Source: CAD feature listing. Evaluate the final solid. Frame: model axes, mm. A direction names the side the tool comes from. Coordinates: 2 decimals unless noted, no trailing zeros. Order: outer loops, then holes, each group sorted by start corner. A loop starts at its lowest first (then second) coordinate and runs counter-clockwise, first axis right, second up. Notation, with made-up numbers: (0.5, 14.5) - (44.5, 14.5) arc R9 cw to (44.5, 25.5) - close; hole circle Ø8 at (38, -21.5). An arc over 180 degrees is marked (long way). One line per question, with ' | ' between items. Start each with the question number.
(1) Contact query for flat-ended pins moving along their axis: P1, Ø5, axis at x = -55.5, z = 10.5, coming from the -Y side; P2, Ø5, axis at x = 1.5, z = -20, coming from the +Y side; P3, Ø8, axis at x = 1.5, z = 20, coming from the -Y side; P4, Ø3, axis at x = -48.5, z = -20, coming from the +Y side. Output: stop coordinate, or through.
(2) Line query: line 1 along X through (y, z) = (22.05, 20); line 2 along X through (y, z) = (8.25, 18.5); line 3 along Z through (x, y) = (51.5, 12.75). Output: solid intervals per line, ascending.
(3) Draft query along Z for faces 5 (the flat face through (1, 15, -33)), 6 (the flat face through (1, 8, 31.2)), 7 (the flat face through (1, 24.25, 0)). Return one class per face: +Z half, -Z half, draft (parallel to the pull), parting line (faces both ways), or undercut.
(4) Section B-B (z = 9.92). Return the cut outline in (x, y), then the cut area to 3 significant figures.
(5) Section A-A (x = -24). Return the cut outline in (y, z), then the cut area to 3 significant figures.
(6) Section C-C (z = 20). Count the separate pieces of the cut face and the enclosed holes in it, then the cut area to 3 significant figures.
(7) Access query for faces 1 (the cylindrical face through (-56.542, 11.694, -5.981)), 2 (the flat face through (40, 21.05, -19)), 3 (the flat face through (-57.7, 8, 2)), 4 (the cylindrical face through (39.94, 17.82, -20.35)). Directions: +Z, -Z, +X, -X, +Y, -Y. A direction counts if a zero-diameter tool reaches every point of the face in a straight line with its end or side. Return the directions, or none.
from build123d import *

# Parameters (mm, degrees)
SKETCH1_W           = 107
SKETCH1_H           = 54
BOSS_EXTRUDE1_DEPTH = 13
CUT_EXTRUDE1_DEPTH  = 2.2
BOSS_EXTRUDE2_DEPTH = 4
FILLET1_R           = 2
SKETCH4_R           = 6
CUT_EXTRUDE2_DEPTH  = 6
CUT_EXTRUDE3_DEPTH  = 6
SKETCH9_R           = 4
SKETCH9_R_2         = 1.6
BOSS_EXTRUDE3_DEPTH = 9.75
SKETCH10_R          = 3
CUT_EXTRUDE5_DEPTH  = 3.2
SKETCH10_3_R        = 1.6
CUT_EXTRUDE6_DEPTH  = 71.13023599


with BuildPart() as part:
    # Sketch1 → Boss-Extrude1 (new body)
    with BuildSketch(Plane(origin=(0, 7.25, 0), x_dir=(1, 0, 0), z_dir=(0, 1, 0))):
        with BuildLine():
            Line((-54.5, -33), (54.5, -33))
            ThreePointArc((54.5, -33), (58.035533906, -31.535533906), (59.5, -28))
            Line((59.5, -28), (59.5, 28))
            ThreePointArc((59.5, 28), (58.035533906, 31.535533906), (54.5, 33))
            Line((54.5, 33), (-54.5, 33))
            ThreePointArc((-54.5, 33), (-58.035533906, 31.535533906), (-59.5, 28))
            Line((-59.5, 28), (-59.5, -28))
            ThreePointArc((-59.5, -28), (-58.035533906, -31.535533906), (-54.5, -33))
        make_face()
        Rectangle(SKETCH1_W, SKETCH1_H, mode=Mode.SUBTRACT)
    extrude(amount=BOSS_EXTRUDE1_DEPTH)

    # Sketch2 → Cut-Extrude1 (cut)
    with BuildSketch(Plane.XZ.offset(-7.25)):
        with BuildLine():
            Line((-52.7, -31.2), (52.7, -31.2))
            ThreePointArc((52.7, -31.2), (56.235533906, -29.735533906), (57.7, -26.2))
            Line((57.7, -26.2), (57.7, 26.2))
            ThreePointArc((57.7, 26.2), (56.235533906, 29.735533906), (52.7, 31.2))
            Line((52.7, 31.2), (-52.7, 31.2))
            ThreePointArc((-52.7, 31.2), (-56.235533906, 29.735533906), (-57.7, 26.2))
            Line((-57.7, 26.2), (-57.7, -26.2))
            ThreePointArc((-57.7, -26.2), (-56.235533906, -29.735533906), (-52.7, -31.2))
        make_face()
    extrude(amount=-CUT_EXTRUDE1_DEPTH, mode=Mode.SUBTRACT)

    # Sketch3 → Boss-Extrude2 (add)
    with BuildSketch(Plane(origin=(0, 20.25, 0), x_dir=(1, 0, 0), z_dir=(0, 1, 0))):
        with BuildLine():
            Line((-54.5, -33), (54.5, -33))
            ThreePointArc((54.5, -33), (58.035533906, -31.535533906), (59.5, -28))
            Line((59.5, -28), (59.5, 28))
            ThreePointArc((59.5, 28), (58.035533906, 31.535533906), (54.5, 33))
            Line((54.5, 33), (-54.5, 33))
            ThreePointArc((-54.5, 33), (-58.035533906, 31.535533906), (-59.5, 28))
            Line((-59.5, 28), (-59.5, -28))
            ThreePointArc((-59.5, -28), (-58.035533906, -31.535533906), (-54.5, -33))
        make_face()
    extrude(amount=BOSS_EXTRUDE2_DEPTH)

    # Fillet1
    fillet1_edges = [part.edges().sort_by_distance(p)[0] for p in [
        (-58.035533906, 24.25, 31.535533906),
        (0, 24.25, 33),
        (58.035533906, 24.25, 31.535533906),
        (59.5, 24.25, 0),
        (58.035533906, 24.25, -31.535533906),
        (0, 24.25, -33),
        (-58.035533906, 24.25, -31.535533906),
        (-59.5, 24.25, 0),
    ]]
    fillet(fillet1_edges, radius=FILLET1_R)

    # Sketch4 → Cut-Extrude2 (cut)
    with BuildSketch(Plane(origin=(59.5, 0, 0), x_dir=(0, 0, -1), z_dir=(1, 0, 0))):
        with Locations((-9.920000153, 7.26879997)):
            Circle(SKETCH4_R)
        with Locations((10.079999847, 7.26879997)):
            Circle(SKETCH4_R)
    extrude(amount=-CUT_EXTRUDE2_DEPTH, mode=Mode.SUBTRACT)

    # Sketch6 → Cut-Extrude3 (cut)
    with BuildSketch(Plane.ZY.offset(59.5)):
        with BuildLine():
            Line((12, 14.25), (6, 14.25))
            ThreePointArc((6, 14.25), (3.878679656, 13.371320344), (3, 11.25))
            Line((3, 11.25), (3, 7.25))
            Line((3, 7.25), (15, 7.25))
            Line((15, 7.25), (15, 11.25))
            ThreePointArc((15, 11.25), (14.121320344, 13.371320344), (12, 14.25))
        make_face()
        with BuildLine():
            Line((-12.769576367, 7.25), (0.569576367, 7.25))
            ThreePointArc((0.569576367, 7.25), (-6.1, 11.695024517), (-12.769576367, 7.25))
        make_face()
    extrude(amount=-CUT_EXTRUDE3_DEPTH, mode=Mode.SUBTRACT)

    # Sketch9 → Boss-Extrude3 (add)
    # profile 1 of 6: a face of its own
    with BuildSketch(Plane(origin=(0, 24.25, 0), x_dir=(1, 0, 0), z_dir=(0, 1, 0))):
        with Locations(Location((-48.5, -20, 0), (0, 0, 270))):
            Circle(SKETCH9_R)
        with Locations(Location((-48.5, -20, 0), (0, 0, 270))):
            Circle(SKETCH9_R_2, mode=Mode.SUBTRACT)
    # profile 2 of 6: a face of its own
    with BuildSketch(Plane(origin=(0, 24.25, 0), x_dir=(1, 0, 0), z_dir=(0, 1, 0))):
        with Locations(Location((1.5, -20, 0), (0, 0, 270))):
            Circle(SKETCH9_R)
        with Locations(Location((1.5, -20, 0), (0, 0, 270))):
            Circle(SKETCH9_R_2, mode=Mode.SUBTRACT)
    # profile 3 of 6: a face of its own
    with BuildSketch(Plane(origin=(0, 24.25, 0), x_dir=(1, 0, 0), z_dir=(0, 1, 0))):
        with Locations(Location((41.5, -20, 0), (0, 0, 270))):
            Circle(SKETCH9_R)
        with Locations(Location((41.5, -20, 0), (0, 0, 270))):
            Circle(SKETCH9_R_2, mode=Mode.SUBTRACT)
    # profile 4 of 6: a face of its own
    with BuildSketch(Plane(origin=(0, 24.25, 0), x_dir=(1, 0, 0), z_dir=(0, 1, 0))):
        with Locations(Location((41.5, 20, 0), (0, 0, 270))):
            Circle(SKETCH9_R)
        with Locations(Location((41.5, 20, 0), (0, 0, 270))):
            Circle(SKETCH9_R_2, mode=Mode.SUBTRACT)
    # profile 5 of 6: a face of its own
    with BuildSketch(Plane(origin=(0, 24.25, 0), x_dir=(1, 0, 0), z_dir=(0, 1, 0))):
        with Locations(Location((1.5, 20, 0), (0, 0, 270))):
            Circle(SKETCH9_R)
        with Locations(Location((1.5, 20, 0), (0, 0, 270))):
            Circle(SKETCH9_R_2, mode=Mode.SUBTRACT)
    # profile 6 of 6: a face of its own
    with BuildSketch(Plane(origin=(0, 24.25, 0), x_dir=(1, 0, 0), z_dir=(0, 1, 0))):
        with Locations(Location((-48.5, 20, 0), (0, 0, 270))):
            Circle(SKETCH9_R)
        with Locations(Location((-48.5, 20, 0), (0, 0, 270))):
            Circle(SKETCH9_R_2, mode=Mode.SUBTRACT)
    extrude(amount=-BOSS_EXTRUDE3_DEPTH)

    # Sketch10 → Cut-Extrude5 (cut)
    with BuildSketch(Plane(origin=(0, 24.25, 0), x_dir=(1, 0, 0), z_dir=(0, 1, 0))):
        with Locations(Location((-48.5, 20, 0), (0, 0, 270))):
            Circle(SKETCH10_R)
        with Locations(Location((1.5, 20, 0), (0, 0, 270))):
            Circle(SKETCH10_R)
        with Locations(Location((41.5, 20, 0), (0, 0, 270))):
            Circle(SKETCH10_R)
        with Locations(Location((41.5, -20, 0), (0, 0, 90))):
            Circle(SKETCH10_R)
        with Locations(Location((1.5, -20, 0), (0, 0, 90))):
            Circle(SKETCH10_R)
        with Locations(Location((-48.5, -20, 0), (0, 0, 90))):
            Circle(SKETCH10_R)
    extrude(amount=-CUT_EXTRUDE5_DEPTH, mode=Mode.SUBTRACT)

    # Sketch10_3 → Cut-Extrude6 (cut, through all)
    with BuildSketch(Plane(origin=(0, 24.25, 0), x_dir=(1, 0, 0), z_dir=(0, 1, 0))):
        with Locations(Location((-48.5, 20, 0), (0, 0, 270))):
            Circle(SKETCH10_3_R)
        with Locations(Location((1.5, 20, 0), (0, 0, 270))):
            Circle(SKETCH10_3_R)
        with Locations(Location((41.5, 20, 0), (0, 0, 270))):
            Circle(SKETCH10_3_R)
        with Locations(Location((41.5, -20, 0), (0, 0, 270))):
            Circle(SKETCH10_3_R)
        with Locations(Location((1.5, -20, 0), (0, 0, 270))):
            Circle(SKETCH10_3_R)
        with Locations(Location((-48.5, -20, 0), (0, 0, 270))):
            Circle(SKETCH10_3_R)
    extrude(amount=-CUT_EXTRUDE6_DEPTH, mode=Mode.SUBTRACT)


solid = part.part
Response values:
1) P1: stops at y = 14.08 | P2: stops at y = 21.05 | P3: stops at y = 14.5 | P4: passes through
2) line 1: x = -59.5 to -51.5, -45.5 to -1.5, 4.5 to 38.5, 44.5 to 59.5 | line 2: x = -59.5 to -57.7, 57.7 to 59.5 | line 3: z = -33 to -27, 27 to 33
3) face 5: -Z half | face 6: undercut | face 7: draft
4) outline: (-59.5, 14.25) - (-53.5, 14.25) - (-53.5, 20.25) - (53.5, 20.25) - (53.5, 13.27) - (59.5, 13.27) - (59.5, 22.25) arc R2 ccw to (57.5, 24.25) - (-57.5, 24.25) arc R2 ccw to (-59.5, 22.25) - close | area: 552 mm²
5) outline: (7.25, -33) - (22.25, -33) arc R2 ccw to (24.25, -31) - (24.25, 31) arc R2 ccw to (22.25, 33) - (7.25, 33) - (7.25, 31.2) - (9.45, 31.2) - (9.45, 27) - (20.25, 27) - (20.25, -27) - (9.45, -27) - (9.45, -31.2) - (7.25, -31.2) - close | area: 400 mm²
6) separate pieces: 4 | enclosed holes: 0 | area: 629 mm²
7) face 1: -X, -Y | face 2: +Y | face 3: -Y | face 4: +Y, -Y
